Here's how the part is built. I have some questions about the finished solid (model axes, mm). A direction names the side the tool comes from. Coordinates: 2 decimals unless noted, no trailing zeros. Write each loop counter-clockwise with the first axis right and the second up, starting at its lowest first coordinate (ties: lowest second). Pieces come first, ordered by that corner, then holes.
(1) Which directions (+Z, -Z, +X, -X, +Y, -Y) give clear straight access to the entire face, cutting with the end or side of a thin tool? Please do faces 1 (the flat face through (15.366, -3, 1)), 2 (the flat face through (14, 1.823, 1)), 3 (the flat face through (-3, 15.366, 1)).
(2) Thinking about a two-plate mould opening in Y: for faces 4 (the flat face through (-14, 1.302, 1)), 5 (the flat face through (-3, -15.366, 1)), 6 (the flat face through (-5.115, 28, 1)), 7 (the cylindrical face through (28.078, -1.805, 1.479)), which applies, released by +Y, released by -Y, zero draft, split by the parting line, or undercut?
(3) For pin 1 Ø0.9 at (y, z) = (-29.5, 2) entering from +X; pin 2 Ø1.3 at (y, z) = (-2.5, 2) entering from -X; pin 3 Ø1.5 at (x, z) = (-25, 2) entering from -Y, each with a flat end and sliding along its axis, tell me the tip position at first contact or that it passes through.
(4) Imagine slicing it at A-A, the plane x = -21.5. List the corners of the cut face in (y, z) for me, plus the area to 3 significant figures.
(5) Please list where these lines run through material, in increasing order: probe 1 along Y at (x, z) = (0, 2); probe 2 along X at (y, z) = (-1, 2); probe 3 along X at (y, z) = (-4.5, 2.4).
(6) Imagine slicing it at B-B, the plane x = 0. List the corners of the cut face in (y, z) for me, plus the area to 3 significant figures.
(7) Imagine slicing it at D-D, the plane z = 1.2. State how many separate pieces and enclosed holes the cut face has, plus the area to 3 significant figures.
```python
from build123d import *

# Parameters (mm, degrees)
F0_R     = 2
F0_R_2   = 11
F1_DEPTH = 3


with BuildPart() as f1:
    # F0 (on Top) → F1 (new body)
    with BuildSketch(Plane.XY):
        with BuildLine():
            Line((-1.822556, 15.366418), (1.301658, 15.366418))
            Line((1.301658, 15.366418), (3.884909, 15.366418))
            ThreePointArc((3.884909, 15.366418), (1.741215, 28.250033), (-5.115091, 39.366418))
            Line((-5.115091, 39.366418), (-5.115091, 15.366418))
            Line((-5.115091, 15.366418), (-1.822556, 15.366418))
        make_face()
        with Locations((0, 21.95785)):
            Circle(F0_R, mode=Mode.SUBTRACT)
        with BuildLine():
            ThreePointArc((-1.822556, 12.366418), (-0.262508, 12.497243), (1.301658, 12.432043))
            Line((1.301658, 12.432043), (1.301658, 15.366418))
            Line((1.301658, 15.366418), (-1.822556, 15.366418))
            Line((-1.822556, 15.366418), (-1.822556, 12.366418))
        make_face()
        with BuildLine():
            ThreePointArc((12.432043, -1.301658), (12.482999, -0.651715), (12.5, 0))
            ThreePointArc((12.5, 0), (12.46656, 0.913722), (12.366418, 1.822556))
            ThreePointArc((12.366418, 1.822556), (8.651264, 9.022507), (1.301658, 12.432043))
            ThreePointArc((1.301658, 12.432043), (-0.262508, 12.497243), (-1.822556, 12.366418))
            ThreePointArc((-1.822556, 12.366418), (-9.022507, 8.651264), (-12.432043, 1.301658))
            ThreePointArc((-12.432043, 1.301658), (-12.497243, -0.262508), (-12.366418, -1.822556))
            ThreePointArc((-12.366418, -1.822556), (-8.651264, -9.022507), (-1.301658, -12.432043))
            ThreePointArc((-1.301658, -12.432043), (0.262508, -12.497243), (1.822556, -12.366418))
            ThreePointArc((1.822556, -12.366418), (9.022507, -8.651264), (12.432043, -1.301658))
        make_face()
        Circle(F0_R_2, mode=Mode.SUBTRACT)
        with BuildLine():
            Line((15.366418, 5.115091), (15.366418, 1.822556))
            Line((15.366418, 1.822556), (15.366418, -1.301658))
            Line((15.366418, -1.301658), (15.366418, -3.884909))
            ThreePointArc((15.366418, -3.884909), (28.250033, -1.741215), (39.366418, 5.115091))
            Line((39.366418, 5.115091), (15.366418, 5.115091))
        make_face()
        with Locations((21.95785, 0)):
            Circle(F0_R, mode=Mode.SUBTRACT)
        with BuildLine():
            Line((1.822556, -15.366418), (1.822556, -12.366418))
            ThreePointArc((1.822556, -12.366418), (0.262508, -12.497243), (-1.301658, -12.432043))
            Line((-1.301658, -12.432043), (-1.301658, -15.366418))
            Line((-1.301658, -15.366418), (1.822556, -15.366418))
        make_face()
        with BuildLine():
            Line((5.115091, -15.366418), (1.822556, -15.366418))
            Line((1.822556, -15.366418), (-1.301658, -15.366418))
            Line((-1.301658, -15.366418), (-3.884909, -15.366418))
            ThreePointArc((-3.884909, -15.366418), (-1.741215, -28.250033), (5.115091, -39.366418))
            Line((5.115091, -39.366418), (5.115091, -15.366418))
        make_face()
        with Locations((0, -21.95785)):
            Circle(F0_R, mode=Mode.SUBTRACT)
        with BuildLine():
            Line((-15.366418, -1.822556), (-15.366418, 1.301658))
            Line((-15.366418, 1.301658), (-15.366418, 3.884909))
            ThreePointArc((-15.366418, 3.884909), (-28.250033, 1.741215), (-39.366418, -5.115091))
            Line((-39.366418, -5.115091), (-15.366418, -5.115091))
            Line((-15.366418, -5.115091), (-15.366418, -1.822556))
        make_face()
        with Locations((-21.95785, 0)):
            Circle(F0_R, mode=Mode.SUBTRACT)
        with BuildLine():
            ThreePointArc((-12.366418, -1.822556), (-12.497243, -0.262508), (-12.432043, 1.301658))
            Line((-12.432043, 1.301658), (-15.366418, 1.301658))
            Line((-15.366418, 1.301658), (-15.366418, -1.822556))
            Line((-15.366418, -1.822556), (-12.366418, -1.822556))
        make_face()
        with BuildLine():
            ThreePointArc((12.366418, 1.822556), (12.46656, 0.913722), (12.5, 0))
            ThreePointArc((12.5, 0), (12.482999, -0.651715), (12.432043, -1.301658))
            Line((12.432043, -1.301658), (15.366418, -1.301658))
            Line((15.366418, -1.301658), (15.366418, 1.822556))
            Line((15.366418, 1.822556), (12.366418, 1.822556))
        make_face()
    extrude(amount=F1_DEPTH)


solid = f1.part
```
Recorded:
1. face 1: +Z, -Z, -Y
1. face 2: +Z, -Z, +Y
1. face 3: +Z, -Z, -X
2. face 4: released by +Y
2. face 5: undercut
2. face 6: zero draft
2. face 7: released by -Y
3. pin 1: stops at x = 5.12
3. pin 2: stops at x = -37.04
3. pin 3: stops at y = -5.12
4. outline: (-5.12, 0) - (-1.95, 0) - (-1.95, 3) - (-5.12, 3) - close; (1.95, 0) - (3.51, 0) - (3.51, 3) - (1.95, 3) - close
4. area: 14.2 mm2
5. probe 1: y = -32.13 to -23.96, -19.96 to -11, 11 to 19.96, 23.96 to 32.13
5. probe 2: x = -33.9 to -23.69, -20.23 to -10.95, 10.95 to 20.23, 23.69 to 30.07
5. probe 3: x = -38.68 to -15.37, -11.66 to -10.04, 10.04 to 11.66
6. outline: (-32.13, 0) - (-23.96, 0) - (-23.96, 3) - (-32.13, 3) - close; (-19.96, 0) - (-11, 0) - (-11, 3) - (-19.96, 3) - close; (11, 0) - (19.96, 0) - (19.96, 3) - (11, 3) - close; (23.96, 0) - (32.13, 0) - (32.13, 3) - (23.96, 3) - close
6. area: 103 mm2
7. separate pieces: 1
7. enclosed holes: 5
7. area: 702 mm2
